Design review of the part built by this model. Coordinates are the model's own, in mm. Coordinates: 2 decimals unless noted, no trailing zeros. Write each loop counter-clockwise with the first axis right and the second up, starting at its lowest first coordinate (ties: lowest second). Pieces come first, ordered by that corner, then holes. Notation, with made-up numbers: (-37, -28) -> (-25, -28) arc R22 cw to (-25, 4) -> close; hole circle Ø3 at (-22.75, 18.25). An arc over 180 degrees is marked (long way). Write item = value, one per line. Start each with the question number.
Autodesk Inventor part; units mm, degrees
ref_plane "YZ Plane" through (0, 0, 0) normal (1, 0, 0) x (0, 1, 0)
ref_plane "XZ Plane" through (0, 0, 0) normal (0, 1, 0) x (-1, 0, 0)
ref_plane "XY Plane" through (0, 0, 0) normal (0, 0, 1) x (1, 0, 0)
sketch "Skizze1" plane through (0, 0, 0) normal (0, 0, 1) x (1, 0, 0)
  line L0 (0, 3) -> (30, 3)
  arc A0 (30, 2.9625) -> (30, 3.0375) centre (30, 3) ccw
  arc A1 (0, 3.0375) -> (0, 2.9625) centre (0, 3) ccw
  line L1 (30, 3) -> (30, 2)
  line L2 (30, 2) -> (77, 2)
  line L3 (77, 2) -> (77, -2)
  line L4 (77, -2) -> (30, -2)
  line L5 (30, -2) -> (30, -3)
  line L6 (0, -3) -> (0, 3)
  circle A2 centre (25, -2) radius 0.6
  line L7 (30, -3) -> (0, -3)
  arc A3 (0, -3.0325) -> (0, -2.9675) centre (0, -3) ccw
  arc A4 (0, 2.9675) -> (0, 3.0325) centre (0, 3) ccw
  arc A5 (-0.0325, 3) -> (0.0325, 3) centre (0, 3) ccw
  arc A6 (29.9675, 3) -> (30.0325, 3) centre (30, 3) ccw
  arc A7 (29.9675, 2) -> (30.0325, 2) centre (30, 2) ccw
  arc A8 (76.9675, 2) -> (77.0325, 2) centre (77, 2) ccw
  arc A9 (77, 2.0325) -> (77, 1.9675) centre (77, 2) ccw
  arc A10 (77, -1.9675) -> (77, -2.0325) centre (77, -2) ccw
  arc A11 (30, -1.9675) -> (30, -2.0325) centre (30, -2) ccw
  arc A12 (30, -2.9675) -> (30, -3.0325) centre (30, -3) ccw
  circle A13 centre (25, 2) radius 0.6
  arc A14 (25, 1.6492) -> (25, 2.3508) centre (25, 2) ccw
  arc A15 (25, 2.3508) -> (25, 1.6492) centre (25, 2) ccw
  arc A16 (25, -2.3508) -> (25, -1.6492) centre (25, -2) ccw
  arc A17 (25, -1.6492) -> (25, -2.3508) centre (25, -2) ccw
  arc A18 (25, 1.6492) -> (25, 2.3508) centre (25, 2) ccw
  arc A19 (25, 2.3508) -> (25, 1.6492) centre (25, 2) ccw
  arc A20 (25, -2.3508) -> (25, -1.6492) centre (25, -2) ccw
  arc A21 (25, -1.6492) -> (25, -2.3508) centre (25, -2) ccw
  circle A22 centre (12.7, 1.27) radius 0.3
  circle A23 centre (12.7, 0) radius 0.3
  circle A24 centre (12.7, -1.27) radius 0.3
  circle A25 centre (13.97, 1.27) radius 0.3
  circle A26 centre (13.97, -1.27) radius 0.3
  arc A27 (35.0325, 0) -> (34.9675, 0) centre (35, 0) ccw
  arc A28 (72.0325, 0) -> (71.9675, 0) centre (72, 0) ccw
  arc A29 (35.0325, 0) -> (34.9675, 0) centre (35, 0) ccw
  arc A30 (30.0325, -2) -> (29.9675, -2) centre (30, -2) ccw
  line L8 (35, 0) -> (72, 0)
  line L9 (12.1968, -0.5032) -> (13.2032, -0.5032)
  line L10 (13.2032, -0.5032) -> (13.2032, 0.5032)
  line L11 (13.2032, 0.5032) -> (12.1968, 0.5032)
  line L12 (12.1968, 0.5032) -> (12.1968, -0.5032)
  line L13 (12.1968, -0.5032) -> (13.2032, -0.5032)
  line L14 (13.2032, -0.5032) -> (13.2032, 0.5032)
  line L15 (13.2032, 0.5032) -> (12.1968, 0.5032)
  line L16 (12.1968, 0.5032) -> (12.1968, -0.5032)
  line L17 (12.0952, -0.6048) -> (13.3048, -0.6048)
  line L18 (13.3048, -0.6048) -> (13.3048, 0.6048)
  line L19 (13.3048, 0.6048) -> (12.0952, 0.6048)
  line L20 (12.0952, 0.6048) -> (12.0952, -0.6048)
  line L21 (12.0952, -0.6048) -> (13.3048, -0.6048)
  line L22 (13.3048, -0.6048) -> (13.3048, 0.6048)
  line L23 (13.3048, 0.6048) -> (12.0952, 0.6048)
  line L24 (12.0952, 0.6048) -> (12.0952, -0.6048)
  line L25 (12.1968, -1.7732) -> (13.2032, -1.7732)
  line L26 (13.2032, -1.7732) -> (13.2032, -0.7668)
  line L27 (13.2032, -0.7668) -> (12.1968, -0.7668)
  line L28 (12.1968, -0.7668) -> (12.1968, -1.7732)
  line L29 (12.1968, -1.7732) -> (13.2032, -1.7732)
  line L30 (13.2032, -1.7732) -> (13.2032, -0.7668)
  line L31 (13.2032, -0.7668) -> (12.1968, -0.7668)
  line L32 (12.1968, -0.7668) -> (12.1968, -1.7732)
  line L33 (12.0952, -1.8748) -> (13.3048, -1.8748)
  line L34 (13.3048, -1.8748) -> (13.3048, -0.6652)
  line L35 (13.3048, -0.6652) -> (12.0952, -0.6652)
  line L36 (12.0952, -0.6652) -> (12.0952, -1.8748)
  line L37 (12.0952, -1.8748) -> (13.3048, -1.8748)
  line L38 (13.3048, -1.8748) -> (13.3048, -0.6652)
  line L39 (13.3048, -0.6652) -> (12.0952, -0.6652)
  line L40 (12.0952, -0.6652) -> (12.0952, -1.8748)
  line L41 (13.4668, 0.7668) -> (14.4732, 0.7668)
  line L42 (14.4732, 0.7668) -> (14.4732, 1.7732)
  line L43 (14.4732, 1.7732) -> (13.4668, 1.7732)
  line L44 (13.4668, 1.7732) -> (13.4668, 0.7668)
  line L45 (13.4668, 0.7668) -> (14.4732, 0.7668)
  line L46 (14.4732, 0.7668) -> (14.4732, 1.7732)
  line L47 (14.4732, 1.7732) -> (13.4668, 1.7732)
  line L48 (13.4668, 1.7732) -> (13.4668, 0.7668)
  line L49 (13.3652, 0.6652) -> (14.5748, 0.6652)
  line L50 (14.5748, 0.6652) -> (14.5748, 1.8748)
  line L51 (14.5748, 1.8748) -> (13.3652, 1.8748)
  line L52 (13.3652, 1.8748) -> (13.3652, 0.6652)
  line L53 (13.3652, 0.6652) -> (14.5748, 0.6652)
  line L54 (14.5748, 0.6652) -> (14.5748, 1.8748)
  line L55 (14.5748, 1.8748) -> (13.3652, 1.8748)
  line L56 (13.3652, 1.8748) -> (13.3652, 0.6652)
  line L57 (13.4668, -1.7732) -> (14.4732, -1.7732)
  line L58 (14.4732, -1.7732) -> (14.4732, -0.7668)
  line L59 (14.4732, -0.7668) -> (13.4668, -0.7668)
  line L60 (13.4668, -0.7668) -> (13.4668, -1.7732)
  line L61 (13.4668, -1.7732) -> (14.4732, -1.7732)
  line L62 (14.4732, -1.7732) -> (14.4732, -0.7668)
  line L63 (14.4732, -0.7668) -> (13.4668, -0.7668)
  line L64 (13.4668, -0.7668) -> (13.4668, -1.7732)
  line L65 (13.3652, -1.8748) -> (14.5748, -1.8748)
  line L66 (14.5748, -1.8748) -> (14.5748, -0.6652)
  line L67 (14.5748, -0.6652) -> (13.3652, -0.6652)
  line L68 (13.3652, -0.6652) -> (13.3652, -1.8748)
  line L69 (13.3652, -1.8748) -> (14.5748, -1.8748)
  line L70 (14.5748, -1.8748) -> (14.5748, -0.6652)
  line L71 (14.5748, -0.6652) -> (13.3652, -0.6652)
  line L72 (13.3652, -0.6652) -> (13.3652, -1.8748)
  line L73 (12.1968, 0.7668) -> (13.2032, 0.7668)
  line L74 (13.2032, 0.7668) -> (13.2032, 1.7732)
  line L75 (13.2032, 1.7732) -> (12.1968, 1.7732)
  line L76 (12.1968, 1.7732) -> (12.1968, 0.7668)
  line L77 (12.1968, 0.7668) -> (13.2032, 0.7668)
  line L78 (13.2032, 0.7668) -> (13.2032, 1.7732)
  line L79 (13.2032, 1.7732) -> (12.1968, 1.7732)
  line L80 (12.1968, 1.7732) -> (12.1968, 0.7668)
  line L81 (12.0952, 0.6652) -> (13.3048, 0.6652)
  line L82 (13.3048, 0.6652) -> (13.3048, 1.8748)
  line L83 (13.3048, 1.8748) -> (12.0952, 1.8748)
  line L84 (12.0952, 1.8748) -> (12.0952, 0.6652)
  line L85 (12.0952, 0.6652) -> (13.3048, 0.6652)
  line L86 (13.3048, 0.6652) -> (13.3048, 1.8748)
  line L87 (13.3048, 1.8748) -> (12.0952, 1.8748)
  line L88 (12.0952, 1.8748) -> (12.0952, 0.6652)
  line L89 (0, 3) -> (30, 3)
  line L90 (30, 3) -> (30, -3)
  line L91 (30, -3) -> (0, -3)
  line L92 (0, -3) -> (0, 3)
  line L93 (30, 2) -> (77, 2)
  line L94 (77, 2) -> (77, -2)
  line L95 (77, -2) -> (30, -2)
  line L96 (30, -2) -> (30, 2)
  line L97 (14.7384, 0.7621) -> (15.7448, 0.7621)
  line L98 (15.7448, 0.7621) -> (15.7448, 1.7685)
  line L99 (15.7448, 1.7685) -> (14.7384, 1.7685)
  line L100 (14.7384, 1.7685) -> (14.7384, 0.7621)
  line L101 (14.7384, 0.7621) -> (15.7448, 0.7621)
  line L102 (15.7448, 0.7621) -> (15.7448, 1.7685)
  line L103 (15.7448, 1.7685) -> (14.7384, 1.7685)
  line L104 (14.6368, 0.6605) -> (15.8464, 0.6605)
  line L105 (15.8464, 0.6605) -> (15.8464, 1.8701)
  line L106 (15.8464, 1.8701) -> (14.6368, 1.8701)
  line L107 (14.6368, 0.6605) -> (15.8464, 0.6605)
  line L108 (15.8464, 0.6605) -> (15.8464, 1.8701)
  line L109 (15.8464, 1.8701) -> (14.6368, 1.8701)
  line L110 (14.6368, 1.8701) -> (14.6368, 0.6605)
  line L111 (14.7384, -1.7779) -> (15.7448, -1.7779)
  line L112 (15.7448, -1.7779) -> (15.7448, -0.7715)
  line L113 (15.7448, -0.7715) -> (14.7384, -0.7715)
  line L114 (14.7384, -1.7779) -> (15.7448, -1.7779)
  line L115 (15.7448, -1.7779) -> (15.7448, -0.7715)
  line L116 (15.7448, -0.7715) -> (14.7384, -0.7715)
  line L117 (14.7384, -0.7715) -> (14.7384, -1.7779)
  line L118 (14.6368, -1.8795) -> (15.8464, -1.8795)
  line L119 (15.8464, -1.8795) -> (15.8464, -0.6699)
  line L120 (15.8464, -0.6699) -> (14.6368, -0.6699)
  line L121 (14.6368, -1.8795) -> (15.8464, -1.8795)
  line L122 (15.8464, -1.8795) -> (15.8464, -0.6699)
  line L123 (15.8464, -0.6699) -> (14.6368, -0.6699)
  line L124 (14.6368, -0.6699) -> (14.6368, -1.8795)
  circle A31 centre (15.24, 1.27) radius 0.3
  circle A32 centre (15.24, -1.2747) radius 0.3
  point P0 (0, 0)
  dimension "d11" = 0.6
  dimension "d12" = 0.6
  dimension "d13" = 0.6
extrude "Extrusion1" add sketch "Skizze1" along normal blind 1 contours L0 A4 L6 | L0 A6 L1 L90 A11 L5 A12 L7 A3 L6 A4 | L0 L1 A6 | A3 L7 L6 | A12 L5 L7 | L90 L5 A11 | L12 L11 L10 L9 | L20 L19 L18 L17 | L28 L27 L26 L25 | L36 L35 L34 L33 | L44 L43 L42 L41 | L52 L51 L50 L49 | L60 L59 L58 L57 | L68 L67 L66 L65 | L76 L75 L74 L73 | L84 L83 L82 L81 | L100 L99 L98 L97 | L110 L106 L105 L104 | L117 L113 L112 L111 | L124 L120 L119 L118 | A31 | A32
extrude "Extrusion4" add sketch "Skizze1" along normal blind 1 contours L2 A7 L90 | L2 A8 L3 A10 L4 A30 L90 A7 | L2 L3 A8 | A30 L4 L90 | L3 L4 A10
extrude "Extrusion5" cut sketch "Skizze1" along normal blind 10 contours A31 | A32
properties part number "PCB"
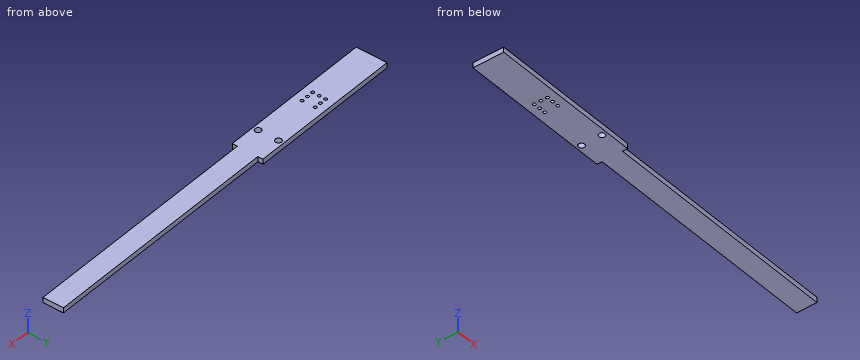
(1) Take a section at A-A, the plane z = 0.15. Count the separate pieces of the cut face and the enclosed holes in it, then the cut area to 3 significant figures.
(2) For line 1 (Y direction, x = 15.24, z = 0.8); line 2 (X direction, y = -1.2, z = 0.1); line 3 (Y direction, x = 25, z = 0.65), list the stretches that pass through material, from the lowest coordinate up.
(3) Take a section at B-B, the plane x = 42.5. State the section outline as (y, z) points, then the cut area to 3 significant figures.
Report:
q1.separate_pieces = 1
q1.enclosed_holes = 9
q1.area = 364 mm2
q2.line_1 = -3 to -1.57, -0.97 to 0.97, 1.57 to 3
q2.line_2 = 0 to 12.41, 12.99 to 13.68, 14.26 to 14.95, 15.53 to 77
q2.line_3 = -3 to -2.6, -1.4 to 1.4, 2.6 to 3
q3.outline = (-2, 0) -> (2, 0) -> (2, 1) -> (-2, 1) -> close
q3.area = 4.00 mm2
